Verification items for the finished model (mm, model axes). Give positions to 0.01 mm unless a question says otherwise; leave off trailing zeros. Write each loop counter-clockwise with the first axis right and the second up, starting at its lowest first coordinate (ties: lowest second). Pieces come first, ordered by that corner, then holes.
from build123d import *

# Parameters (mm, degrees)
SKETCH1_W           = 100
SKETCH1_H           = 20
SKETCH1_R           = 3.3
BOSS_EXTRUDE1_DEPTH = 3.175


with BuildPart() as part:
    # Sketch1 → Boss-Extrude1 (new, symmetric)
    with BuildSketch(Plane.XY):
        Rectangle(SKETCH1_W, SKETCH1_H)
        with Locations((-40, 0)):
            Circle(SKETCH1_R, mode=Mode.SUBTRACT)
        with Locations(Location((40, 0, 0), (0, 0, 180))):
            Circle(SKETCH1_R, mode=Mode.SUBTRACT)
    extrude(amount=BOSS_EXTRUDE1_DEPTH, both=True)


solid = part.part
Item 1: Sectioned sample at A-A on y = 0. Record the cut outline in (x, z) (3 decimals), then the cut area to 3 significant figures.
Answer key:
outline: (-50, -3.175) - (-43.3, -3.175) - (-43.3, 3.175) - (-50, 3.175) - close; (-36.7, -3.175) - (36.7, -3.175) - (36.7, 3.175) - (-36.7, 3.175) - close; (43.3, -3.175) - (50, -3.175) - (50, 3.175) - (43.3, 3.175) - close
area: 551 mm2
Item 2: Scan lines: line 1 along X through (y, z) = (1.75, -3); line 2 along X through (y, z) = (-1.25, -2); line 3 along Y through (x, z) = (-40, 0.25). Record each from-to range of solid material in increasing order.
Answer key:
line 1: x = -50 to -42.8, -37.2 to 37.2, 42.8 to 50
line 2: x = -50 to -43.05, -36.95 to 36.95, 43.05 to 50
line 3: y = -10 to -3.3, 3.3 to 10
Item 3: Sectioned sample at C-C on z = -1.25. Record the cut outline in (x, y).
Answer key:
outline: (-50, -10) - (50, -10) - (50, 10) - (-50, 10) - close; hole circle Ø6.6 at (-40, 0); hole circle Ø6.6 at (40, 0)
Item 4: Release check for a two-part mould opening along X. For faces 1 (the face through (42.619, 2.008, -0.044)), 2 (the face through (-1, 0, 3.175)), 3 (the face through (-50, 0, 0)), 4 (the face through (-42.619, -2.008, -0.044)) record: released by +X, released by -X, zero draft, split by the parting line, or undercut.
Answer key:
face 1: undercut
face 2: zero draft
face 3: released by -X
face 4: undercut
Item 5: Sectioned sample at D-D on x = 42. Record the cut outline in (y, z) (3 decimals).
Answer key:
outline: (-10, -3.175) - (-2.625, -3.175) - (-2.625, 3.175) - (-10, 3.175) - close; (2.625, -3.175) - (10, -3.175) - (10, 3.175) - (2.625, 3.175) - close
Item 6: Sectioned sample at B-B on x = -40. Record the cut outline in (y, z) (3 decimals), then the cut area to 3 significant figures.
Answer key:
outline: (-10, -3.175) - (-3.3, -3.175) - (-3.3, 3.175) - (-10, 3.175) - close; (3.3, -3.175) - (10, -3.175) - (10, 3.175) - (3.3, 3.175) - close
area: 85.1 mm2
